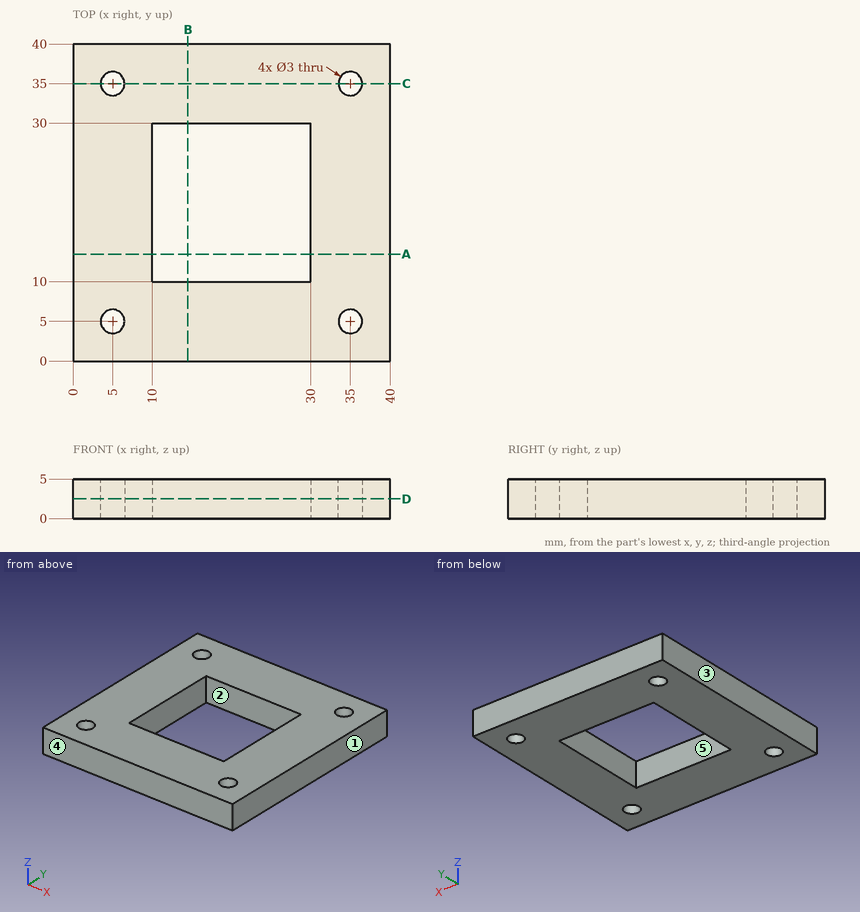
Verification items for this drawing (mm, ordinates from the low corner). A direction names the side the tool comes from. Coordinates: 2 decimals unless noted, no trailing zeros. Loops run counter-clockwise (first coordinate to the right, second up) from the corner with the lowest first, then second, coordinate; pieces in that order, holes last. Notation, with made-up numbers: (40, 40.25) - (63, 40.25) arc R20 ccw to (63, 51.25) - close; hole circle Ø4 at (10, -29.75). An arc over 180 degrees is marked (long way). Use one line per item in the form item = value. Start each with the question number.
Item 1: Mould release check, pull along X, two halves, no side actions. Record for the marked faces 3, 4 and 5: +X half, -X half, draft (parallel to the pull), parting line (faces both ways), or undercut.
Item 2: Section check C-C, the plane y = 35. Enter the section's corners in (x, z), and give its area (3 significant figures).
Item 3: Thickness scan on probe 1 along Y at (x, z) = (5, 1.8); probe 2 along Y at (x, z) = (27.5, 4.2). Record the ranges inside material, lowest first.
Item 4: Section check D-D, the plane z = 2.5. Enter the section's corners in (x, y), and give its area (3 significant figures).
Item 5: Gauge pin test, flat end, axial feed: pin 1 (1.8 mm diameter, centred on x = 5, y = 5, fed in from -Z). Record the tip position at first contact, or that the pin passes through.
Item 6: Section check A-A, the plane y = 13.5. Enter the section's corners in (x, z), and give its area (3 significant figures).
Item 7: Tool access check on the marked faces 1 and 2. Record the directions out of +Z, -Z, +X, -X, +Y, -Y that give a thin tool (end or side, any length) a straight path to the whole face; none if there is none.
Computed:
q1.face_3 = -X half
q1.face_4 = draft
q1.face_5 = undercut
q2.outline = (0, 0) - (3.5, 0) - (3.5, 5) - (0, 5) - close; (6.5, 0) - (33.5, 0) - (33.5, 5) - (6.5, 5) - close; (36.5, 0) - (40, 0) - (40, 5) - (36.5, 5) - close
q2.area = 170 mm2
q3.probe_1 = 0 to 3.5, 6.5 to 33.5, 36.5 to 40
q3.probe_2 = 0 to 10, 30 to 40
q4.outline = (0, 0) - (40, 0) - (40, 40) - (0, 40) - close; hole circle Ø3 at (5, 5); hole circle Ø3 at (5, 35); hole (10, 10) - (30, 10) - (30, 30) - (10, 30) - close; hole circle Ø3 at (35, 5); hole circle Ø3 at (35, 35)
q4.area = 1,170 mm2
q5.pin_1 = through
q6.outline = (0, 0) - (10, 0) - (10, 5) - (0, 5) - close; (30, 0) - (40, 0) - (40, 5) - (30, 5) - close
q6.area = 100 mm2
q7.face_1 = +Z, -Z, +X, +Y, -Y
q7.face_2 = +Z, -Z
